```python
from build123d import *

# Parameters (mm, degrees)
PAD_DEPTH       = 10
SKETCH001_R     = 1.6
POCKET_DEPTH    = 25.251
POCKET002_DEPTH = 5
SKETCH005_W     = 15.25
SKETCH005_H     = 16
POCKET003_DEPTH = 15
POCKET004_DEPTH = 2.5


with BuildPart() as part:
    # Sketch → Pad (new body, symmetric)
    with BuildSketch(Plane.XY):
        with BuildLine():
            ThreePointArc((-17.587282, -6.5), (-1.951346, -18.648183), (15.860722, -10))
            Line((67.5, -10), (15.860722, -10))
            ThreePointArc((67.5, -10), (87.5, 0), (67.5, 10))
            Line((67.5, 10), (15.860722, 10))
            ThreePointArc((15.860722, 10), (0.915927, 18.727615), (-14.809203, 11.5))
            Line((-32.587282, 11.5), (-14.809203, 11.5))
            Line((-32.587282, 1.5), (-32.587282, 11.5))
            Line((-13.667937, 1.5), (-32.587282, 1.5))
            ThreePointArc((-13.667937, -1.5), (13.75, 0), (-13.667937, 1.5))
            Line((-32.587282, -1.5), (-13.667937, -1.5))
            Line((-32.587282, -6.5), (-32.587282, -1.5))
            Line((-17.587282, -6.5), (-32.587282, -6.5))
        make_face()
        with BuildLine():
            ThreePointArc((68, -3.872983), (75, -8), (82, -3.872983))
            Line((82, 3.872983), (82, -3.872983))
            ThreePointArc((82, 3.872983), (75, 8), (68, 3.872983))
            Line((68, 3.872983), (68, -3.872983))
        make_face(mode=Mode.SUBTRACT)
    extrude(amount=PAD_DEPTH, both=True)

    # Sketch001 (on Face1 of Pad) → Pocket (cut, through all)
    with BuildSketch(Plane.XZ.offset(6.5)):
        with Locations((-24.684659, 0)):
            Circle(SKETCH001_R)
    extrude(amount=-POCKET_DEPTH, mode=Mode.SUBTRACT)

    # Sketch003 → Pocket002 (cut)
    with BuildSketch(Plane.XZ.offset(12.5)):
        Polygon((100.061388, 3.464102), (97.061388, 1.732051), (97.061388, -1.732051), (100.061388, -3.464102), (103.061388, -1.732051), (103.061388, 1.732051), align=None)
    extrude(amount=-POCKET002_DEPTH, mode=Mode.SUBTRACT)

    # Sketch005 → Groove (revolve, cut)
    with BuildSketch(Plane.YZ):
        with Locations((7.625, 0)):
            Rectangle(SKETCH005_W, SKETCH005_H)
    revolve(axis=Axis((0, 0, 0), (0, 0, 1)), mode=Mode.SUBTRACT)

    # Sketch006 (on Face3 of Groove) → Pocket003 (cut)
    with BuildSketch(Plane(origin=(0, 0, -10), x_dir=(1, 0, 0), z_dir=(0, 0, -1))):
        with BuildLine():
            ThreePointArc((67.5, -10), (87.5, 0), (67.5, 10))
            Line((67.5, 10), (62.5, 10))
            Line((62.5, -10), (62.5, 10))
            Line((67.5, -10), (62.5, -10))
        make_face()
    extrude(amount=-POCKET003_DEPTH, mode=Mode.SUBTRACT)

    # Sketch007 (on Face12 of Pocket003) → Pocket004 (cut)
    with BuildSketch(Plane(origin=(0, 11.5, 0), x_dir=(-1, 0, 0), z_dir=(0, 1, 0))):
        Polygon((24.684659, 3.319764), (21.809659, 1.659882), (21.809659, -1.659882), (24.684659, -3.319764), (27.559659, -1.659882), (27.559659, 1.659882), align=None)
    extrude(amount=-POCKET004_DEPTH, mode=Mode.SUBTRACT)


solid = part.part
```
Geometry: final body of the model. Coordinates: model frame, mm. A direction names the side the tool comes from. Round coordinates to 2 decimals unless told otherwise and drop trailing zeros. Loops run counter-clockwise (first coordinate to the right, second up) from the corner with the lowest first, then second, coordinate; pieces in that order, holes last.
Item 1: Section C-C, the plane z = -6.5. Output: boundary loops of the cut face in (x, y), plus the area to 3 significant figures.
Checked values:
outline: (-32.59, -6.5) - (-17.59, -6.5) arc R18.75 ccw to (15.86, -10) - (62.5, -10) - (62.5, 10) - (15.86, 10) arc R18.75 ccw to (-14.81, 11.5) - (-32.59, 11.5) - (-32.59, 1.5) - (-15.18, 1.5) arc R15.25 cw (long way) to (-15.18, -1.5) - (-32.59, -1.5) - close
area: 1,480 mm2
Item 2: Section A-A, the plane x = 0. Output: boundary loops of the cut face in (y, z).
Checked values:
outline: (-18.75, -10) - (-13.75, -10) - (-13.75, -8) - (-15.25, -8) - (-15.25, 8) - (-13.75, 8) - (-13.75, 10) - (-18.75, 10) - close; (13.75, -10) - (18.75, -10) - (18.75, 10) - (13.75, 10) - (13.75, 8) - (15.25, 8) - (15.25, -8) - (13.75, -8) - close
Item 3: Section B-B, the plane y = 6.5. Output: boundary loops of the cut face in (x, z).
Checked values:
outline: (-32.59, -10) - (-12.12, -10) - (-12.12, -8) - (-13.8, -8) - (-13.8, 8) - (-12.12, 8) - (-12.12, 10) - (-32.59, 10) - close; (12.12, -10) - (62.5, -10) - (62.5, 5) - (70.34, 5) - (70.34, 10) - (12.12, 10) - (12.12, 8) - (13.8, 8) - (13.8, -8) - (12.12, -8) - close; (79.66, 5) - (85.68, 5) - (85.68, 10) - (79.66, 10) - close; hole circle Ø3.2 at (-24.68, 0)
Item 4: Contact query for flat-ended pins moving along their axis: P1, Ø6, axis at x = 48, z = -1.5, coming from the -Y side; P2, Ø8, axis at x = -15, z = -7.5, coming from the -Y side; P3, Ø1.7, axis at x = -26, z = -0.5, coming from the +Y side. Output: stop coordinate, or through.
Checked values:
P1: stops at y = -10
P2: stops at y = -15.18
P3: stops at y = 9
Item 5: Section D-D, the plane y = 0. Output: boundary loops of the cut face in (x, z), plus the area to 3 significant figures.
Checked values:
outline: (13.75, -10) - (62.5, -10) - (62.5, 5) - (68, 5) - (68, 10) - (13.75, 10) - (13.75, 8) - (15.25, 8) - (15.25, -8) - (13.75, -8) - close; (82, 5) - (87.5, 5) - (87.5, 10) - (82, 10) - close
area: 1,010 mm2
Item 6: Line query: L1, parallel to Z at x = 10, y = 10; L2, parallel to Y at x = 0, z = -2.25; L3, parallel to Y at x = 0, z = -9.4. Output: solid intervals per line, ascending.
Checked values:
L1: z = -10 to -8, 8 to 10
L2: y = -18.75 to -15.25, 15.25 to 18.75
L3: y = -18.75 to -13.75, 13.75 to 18.75
Item 7: Mould query, pull axis Z, two halves, no side actions, for faces 1 (the flat face through (25, 0, -10)), 2 (the flat face through (-27, -6.5, 0)), 3 (the flat face through (-27.56, 10, 0)). Classes: released by +Z, released by -Z, zero draft, split by the parting line, or undercut.
Checked values:
face 1: released by -Z
face 2: zero draft
face 3: undercut
Item 8: Reachability of faces 4 (the flat face through (2, 14, 8)), 5 (the flat face through (-23.23, 10.27, -2.48)), 6 (the flat face through (-23, 1.5, -2)), 7 (the flat face through (42, -10, 0)) from +Z, -Z, +X, -X, +Y, -Y: full face, straight path, thin tool, end or side. Return the list, or none.
Checked values:
face 4: none
face 5: +Y
face 6: +Z, -Z, -X
face 7: +Z, -Z, -Y
